Check sheet for the drawn part. Datum: minimum x, y, z corner. Units: mm. A direction names the side the tool comes from. Round coordinates to 2 decimals unless told otherwise and drop trailing zeros. Order: outer loops, then holes, each group sorted by start corner. A loop starts at its lowest first (then second) coordinate and runs counter-clockwise, first axis right, second up.
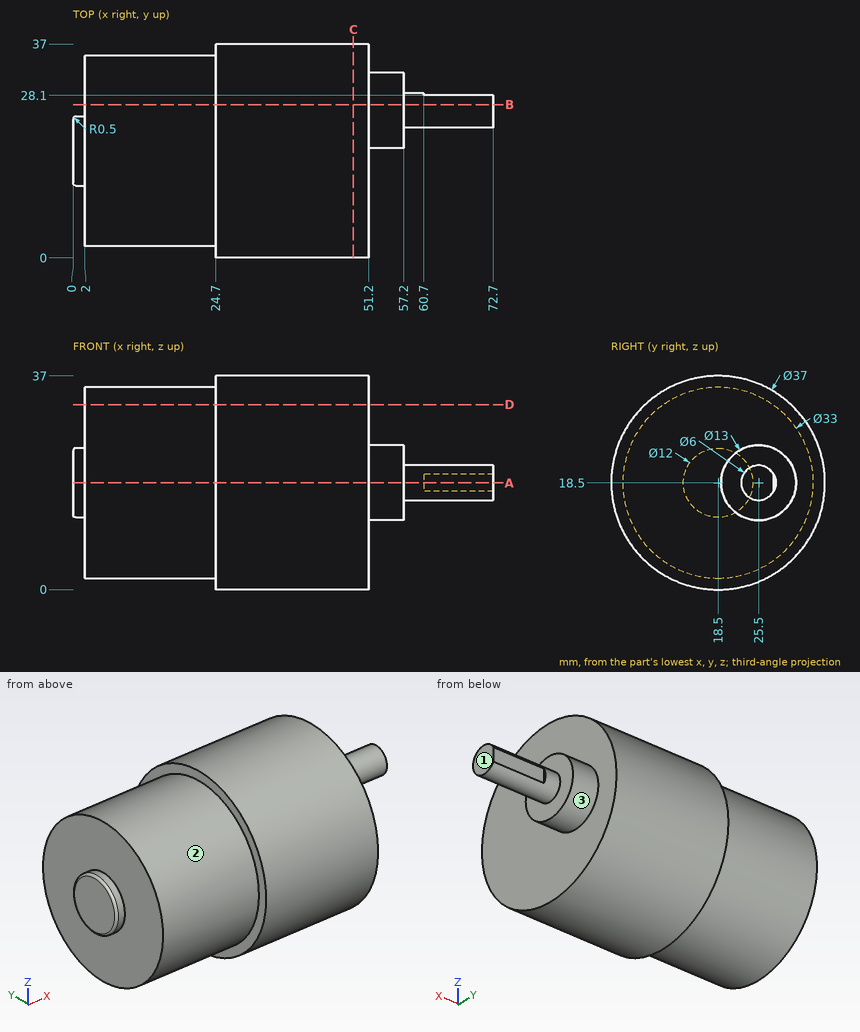
1) Sectioned sample at B-B on y = 26.5. Record the cut outline in (x, z), and give its area (3 significant figures).
2) Set-up check for the marked faces 1, 2 and 3: record each of +Z, -Z, +X, -X, +Y, -Y from which the full face is reachable in a straight line by a thin tool's end or side.
3) Scan lines: line 1 (Y direction, x = 47.5, z = 18.5); line 2 (X direction, y = 18.5, z = 21.5); line 3 (X direction, y = 15.5, z = 31). Record each from-to range of solid material in increasing order.
4) Sectioned sample at A-A on z = 18.5. Record the cut outline in (x, y), and give its area (3 significant figures).
5) Sectioned sample at C-C on x = 48.5. Record the cut outline in (y, z).
6) Gauge pin test, flat ends, axial feed: pin 1 (2 mm diameter, centred on x = 23, z = 7.5, fed in from -Y); pin 2 (12 mm diameter, centred on x = 57.5, z = 9, fed in from -Y); pin 3 (1.5 mm diameter, centred on x = 67.5, z = 18, fed in from +Y). Record the tip position at first contact, or that the pin passes through.
7) Sectioned sample at D-D on z = 32. Record the cut outline in (x, y).
Values found:
1. outline: (2, 4.07) - (24.7, 4.07) - (24.7, 1.82) - (51.2, 1.82) - (51.2, 12.08) - (57.2, 12.08) - (57.2, 15.67) - (72.7, 15.67) - (72.7, 21.33) - (57.2, 21.33) - (57.2, 24.92) - (51.2, 24.92) - (51.2, 35.18) - (24.7, 35.18) - (24.7, 32.93) - (2, 32.93) - close
1. area: 1,700 mm2
2. face 1: +Z, -Z, +X, +Y, -Y
2. face 2: -X
2. face 3: +X
3. line 1: y = 0 to 37
3. line 2: x = 0 to 51.2
3. line 3: x = 2 to 51.2
4. outline: (0, 13) arc R0.5 ccw to (0.5, 12.5) - (2, 12.5) - (2, 2) - (24.7, 2) - (24.7, 0) - (51.2, 0) - (51.2, 19) - (57.2, 19) - (57.2, 22.5) - (72.7, 22.5) - (72.7, 28.1) - (60.7, 28.1) - (60.7, 28.5) - (57.2, 28.5) - (57.2, 32) - (51.2, 32) - (51.2, 37) - (24.7, 37) - (24.7, 35) - (2, 35) - (2, 24.5) - (0.5, 24.5) arc R0.5 ccw to (0, 24) - close
4. area: 1,920 mm2
5. outline: circle Ø37 at (18.5, 18.5)
6. pin 1: stops at y = 5.38
6. pin 2: stops at y = 20.03
6. pin 3: stops at y = 28.1
7. outline: (2, 9.01) - (24.7, 9.01) - (24.7, 5.85) - (51.2, 5.85) - (51.2, 31.15) - (24.7, 31.15) - (24.7, 27.99) - (2, 27.99) - close
